Input: dimensioned drawing with shaded views. Units: mm. Origin: part minimum x, y, z. A direction names the side the tool comes from. Round coordinates to 2 decimals unless told otherwise and drop trailing zeros. Loops run counter-clockwise (first coordinate to the right, second up) from the corner with the lowest first, then second, coordinate; pieces in that order, holes last. Notation, with made-up numbers: (30.25, 74) - (78.25, 74) arc R23 ccw to (78.25, 95) - close; hole circle Ø1 at (-27, 9). An arc over 180 degrees is marked (long way). Write each question's results on one line, items separated by ' | '.
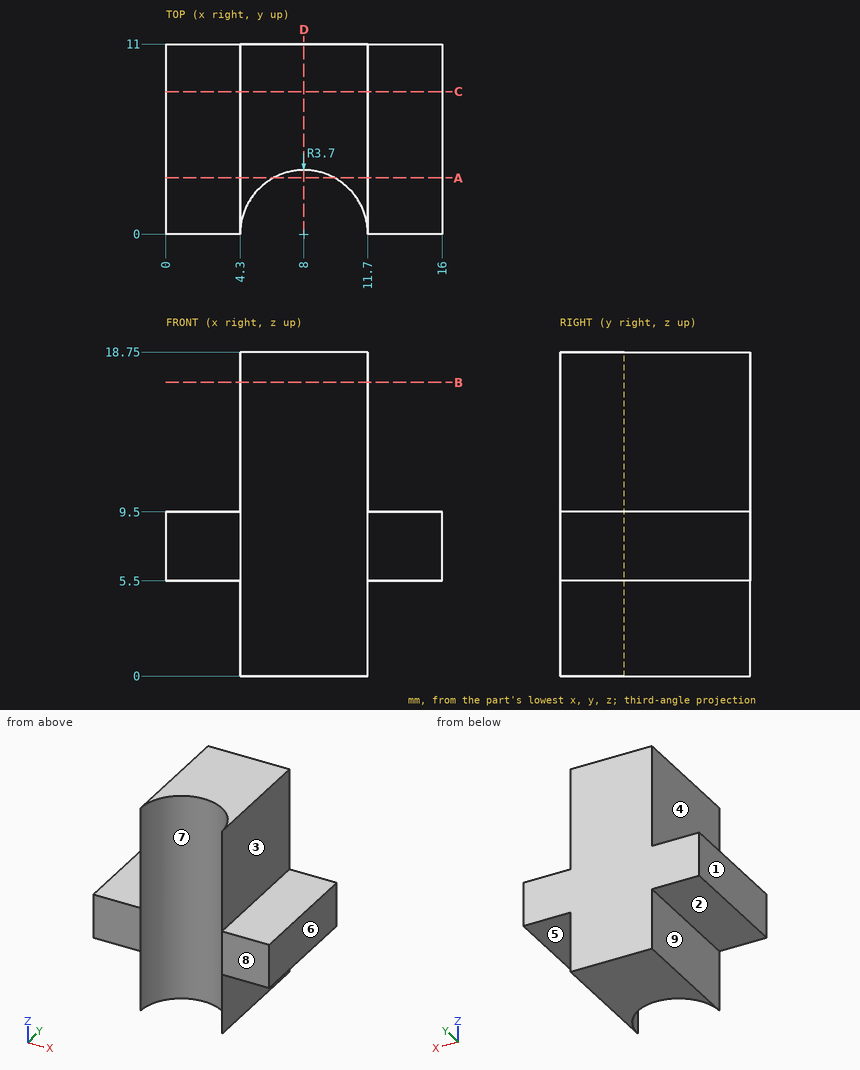
1. Section query C-C, the plane y = 8.25. Output: boundary loops of the cut face in (x, z).
Answer:
outline: (0, 5.5) - (4.3, 5.5) - (4.3, 0) - (11.7, 0) - (11.7, 5.5) - (16, 5.5) - (16, 9.5) - (11.7, 9.5) - (11.7, 18.75) - (4.3, 18.75) - (4.3, 9.5) - (0, 9.5) - close
2. Mould query, pull axis X, two halves, no side actions, for the marked faces 6, 7, 8 and 9. Classes: pulls with the +X half, pulls with the -X half, needs draft (parallel to the pull), parting line crosses it, or undercut.
Answer:
face 6: pulls with the +X half | face 7: undercut | face 8: needs draft | face 9: pulls with the -X half
3. Line query: line 1 (Z direction, x = 3.75, y = 4); line 2 (X direction, y = 8.5, z = 16); line 3 (Y direction, x = 5.75, z = 12.25). Output: solid intervals per line, ascending. Write a range as [from, to].
Answer:
line 1: [5.5, 9.5] | line 2: [4.3, 11.7] | line 3: [2.94, 11]
4. Section query B-B, the plane z = 17. Output: boundary loops of the cut face in (x, y), plus the area to 3 significant figures.
Answer:
outline: (4.3, 0) arc R3.7 cw to (11.7, 0) - (11.7, 11) - (4.3, 11) - close | area: 59.9 mm^2
5. Set-up query: the marked faces 1, 2, 3, 4 and 5. Return all of +Z, -Z, +X, -X, +Y, -Y with unobstructed straight access to the full face (end or side cutting, diameter ignored); none if empty.
Answer:
face 1: +Z, -Z, -X, +Y, -Y | face 2: -Z, -X, +Y, -Y | face 3: +Z, +X, +Y, -Y | face 4: +Z, -X, +Y, -Y | face 5: -Z, +X, +Y, -Y
6. Contact query for flat-ended pins moving along their axis: pin 1 (1.3 mm diameter, centred on x = 14.5, y = 6.5, fed in from -Z); pin 2 (1.3 mm diameter, centred on x = 1, y = 7.5, fed in from +Z); pin 3 (2.5 mm diameter, centred on y = 6.5, z = 1.5, fed in from -X). Output: stop coordinate, or through.
Answer:
pin 1: z = 5.5 | pin 2: z = 9.5 | pin 3: x = 4.3
7. Section query A-A, the plane y = 3.25. Output: boundary loops of the cut face in (x, z), plus the area to 3 significant figures.
Answer:
outline: (0, 5.5) - (4.3, 5.5) - (4.3, 0) - (6.23, 0) - (6.23, 18.75) - (4.3, 18.75) - (4.3, 9.5) - (0, 9.5) - close; (9.77, 0) - (11.7, 0) - (11.7, 5.5) - (16, 5.5) - (16, 9.5) - (11.7, 9.5) - (11.7, 18.75) - (9.77, 18.75) - close | area: 107 mm^2
8. Section query D-D, the plane x = 8. Output: boundary loops of the cut face in (y, z).
Answer:
outline: (3.7, 0) - (11, 0) - (11, 18.75) - (3.7, 18.75) - close
